Autodesk Inventor part; units mm, degrees
ref_plane "YZ Plane" through (0, 0, 0) normal (1, 0, 0) x (0, 1, 0)
ref_plane "XZ Plane" through (0, 0, 0) normal (0, 1, 0) x (-1, 0, 0)
ref_plane "XY Plane" through (0, 0, 0) normal (0, 0, 1) x (1, 0, 0)
sketch "Skizze2" plane through (0, 0, 0) normal (0, 0, 1) x (1, 0, 0)
  line L0 (-26, 0) -> (156, 0)
  line L1 (0, -16) -> (0, 96)
  line L2 (0, 0) -> (130, 0)
  line L3 (130, 0) -> (130, 80)
  line L4 (130, 80) -> (0, 80)
  line L5 (0, 80) -> (0, 0)
  point P0 (0, 80)
  dimension "d0" = 80
  dimension "d1" = 130
extrude "Extrusion1" add sketch "Skizze2" along normal blind 15
sketch "Skizze3" plane through (0, 0, 15) normal (0, 0, 1) x (1, 0, 0)
  line L0 (5, 75) -> (125, 75)
  line L1 (125, 75) -> (125, 5)
  line L2 (125, 5) -> (5, 5)
  line L3 (5, 5) -> (5, 75)
  line L4 (130, 80) -> (0, 80)
  line L5 (130, 0) -> (130, 80)
  line L6 (0, 0) -> (130, 0)
  line L7 (0, 80) -> (0, 0)
  dimension "d4" = 5
  dimension "d5" = 5
  dimension "d6" = 5
  dimension "d7" = 5
extrude "Extrusion2" cut sketch "Skizze3" against normal blind 3 contours L0 L1 L2 L3
fillet "Rundung1" radius 3 4 edges at (65, 75, 15) (5, 40, 15) (65, 5, 15) (125, 40, 15)
properties part number "Display_Dummy"
Source: CAD feature listing. Evaluate the final solid. Frame: model axes, mm. A direction names the side the tool comes from. Round coordinates to 2 decimals unless told otherwise and drop trailing zeros. Use a Markdown table: item, result. Add a question column.
1. Mould query, pull axis X, two halves, no side actions, for faces 1 (the flat face through (65, 79, 15)), 2 (the flat face through (0, 39, 7)), 3 (the cylindrical face through (4.1, 40.53, 14.14)). Classes: pulls with the +X half, pulls with the -X half, needs draft (parallel to the pull), parting line crosses it, or undercut.
2. Contact query for a flat-ended pin moving along its axis: P1, Ø21, axis at x = 50.5, y = 31, coming from the +Z side. Output: stop coordinate, or through.
3. Reachability of faces 4 (the flat face through (64, 0, 7)), 5 (the cylindrical face through (64.12, 4.1, 14.14)) from +Z, -Z, +X, -X, +Y, -Y: full face, straight path, thin tool, end or side. Return the list, or none.
4. Line query: line 1 (Z direction, x = 108.5, y = 32.5); line 2 (Y direction, x = 84, z = 14); line 3 (X direction, y = 67, z = 14.25). Output: solid intervals per line, ascending.
Reported:
| question | item | result |
|---|---|---|
| 1 | face 1 | needs draft |
| 1 | face 2 | pulls with the -X half |
| 1 | face 3 | undercut |
| 2 | P1 | stops at z = 12 |
| 3 | face 4 | +Z, -Z, +X, -X, -Y |
| 3 | face 5 | +Z |
| 4 | line 1 | z = 0 to 12 |
| 4 | line 2 | y = 0 to 4.24, 75.76 to 80 |
| 4 | line 3 | x = 0 to 3.98, 126.02 to 130 |
